from build123d import *

# Parameters (mm, degrees)
SALIENTE_EXTRUIR1_DEPTH    = 5
SALIENTE_EXTRUIR4_DEPTH    = 15
SALIENTE_EXTRUIR6_DEPTH    = 3
SALIENTE_EXTRUIR10_DEPTH   = 1
CROQUIS8_W                 = 24
CROQUIS8_H                 = 2
SALIENTE_EXTRUIR8_DEPTH    = 6
CROQUIS18_W                = 24
CROQUIS18_H                = 2
SALIENTE_EXTRUIR14_DEPTH   = 6
CROQUIS12_R                = 1.75
CORTAR_EXTRUIR1_DEPTH      = 29
CORTAR_EXTRUIR1_DEPTH_BACK = 3
CHAFL_N4_SIZE              = 7
CHAFL_N5_SIZE              = 10
REDONDEO1_R                = 3


with BuildPart() as part:
    # Croquis1 → Saliente-Extruir1 (new body)
    with BuildSketch(Plane.XY):
        with BuildLine():
            Line((0, 0), (24, 0))
            ThreePointArc((24, 0), (32, 8), (40, 0))
            Line((40, 0), (46, 0))
            Line((46, 0), (46, 12))
            Line((46, 12), (73, 12))
            Line((73, 12), (73, 0))
            Line((73, 0), (79, 0))
            Line((79, 0), (79, 30))
            Line((79, 30), (0, 30))
            Line((0, 30), (0, 0))
        make_face()
    extrude(amount=SALIENTE_EXTRUIR1_DEPTH)

    # Croquis4 → Saliente-Extruir4 (add)
    with BuildSketch(Plane.XY.offset(5)):
        Polygon((0, 30), (0, 0), (3, 0), (3, 27), (76, 27), (76, 0), (79, 0), (79, 30), align=None)
    extrude(amount=SALIENTE_EXTRUIR4_DEPTH)

    # Croquis6 → Saliente-Extruir6 (add)
    with BuildSketch(Plane.XY.offset(20)):
        with BuildLine():
            Line((0, 0), (0, 30))
            Line((0, 30), (79, 30))
            Line((79, 30), (79, 0))
            Line((79, 0), (40, 0))
            ThreePointArc((40, 0), (32, 8), (24, 0))
            Line((24, 0), (0, 0))
        make_face()
    extrude(amount=SALIENTE_EXTRUIR6_DEPTH)

    # Croquis13 → Saliente-Extruir10 (add)
    with BuildSketch(Plane(origin=(0, 0, 0), x_dir=(-1, 0, 0), z_dir=(0, 0, -1))):
        with BuildLine():
            Line((-79, 30), (-79, 0))
            Line((-79, 0), (-73, 0))
            Line((-73, 0), (-73, 12))
            Line((-73, 12), (-46, 12))
            Line((-46, 12), (-46, 0))
            Line((-46, 0), (-40, 0))
            Line((-40, 0), (-38, 0))
            ThreePointArc((-38, 0), (-32, 6), (-26, 0))
            Line((-26, 0), (0, 0))
            Line((0, 0), (0, 30))
            Line((0, 30), (-79, 30))
        make_face()
    extrude(amount=SALIENTE_EXTRUIR10_DEPTH)

    # Croquis8 → Saliente-Extruir8 (add)
    with BuildSketch(Plane(origin=(79, 0, 0), x_dir=(0, 0, -1), z_dir=(1, 0, 0))):
        with Locations((-11, 1)):
            Rectangle(CROQUIS8_W, CROQUIS8_H)
    extrude(amount=SALIENTE_EXTRUIR8_DEPTH)

    # Croquis18 → Saliente-Extruir14 (add)
    with BuildSketch(Plane.ZY):
        with Locations((11, 1)):
            Rectangle(CROQUIS18_W, CROQUIS18_H)
    extrude(amount=SALIENTE_EXTRUIR14_DEPTH)

    # Croquis12 → Cortar-Extruir1 (cut, two sides)
    with BuildSketch(Plane(origin=(0, 2, 0), x_dir=(1, 0, 0), z_dir=(0, 1, 0))) as cortar_extruir1_sk:
        with Locations((-3, -5)):
            Circle(CROQUIS12_R)
        with Locations((-3, -17)):
            Circle(CROQUIS12_R)
        with Locations((82, -17)):
            Circle(CROQUIS12_R)
        with Locations((82, -5)):
            Circle(CROQUIS12_R)
    extrude(amount=CORTAR_EXTRUIR1_DEPTH, mode=Mode.SUBTRACT)
    extrude(cortar_extruir1_sk.sketch, amount=-CORTAR_EXTRUIR1_DEPTH_BACK, mode=Mode.SUBTRACT)

    # Chaflán4
    chafl_n4_edges = [part.edges().sort_by_distance(p)[0] for p in [
        (3, 27, 12.5),
        (76, 27, 12.5),
    ]]
    chamfer(chafl_n4_edges, length=CHAFL_N4_SIZE)

    # Chaflán5
    chafl_n5_edges = [part.edges().sort_by_distance(p)[0] for p in [
        (0, 30, 11),
        (79, 30, 11),
    ]]
    chamfer(chafl_n5_edges, length=CHAFL_N5_SIZE)

    # Redondeo1
    redondeo1_edges = [part.edges().sort_by_distance(p)[0] for p in [
        (73, 12, 2),
        (46, 12, 2),
    ]]
    fillet(redondeo1_edges, radius=REDONDEO1_R)


solid = part.part
The listing builds one solid part. Answer for the finished solid, in the listing's coordinates (mm). A direction names the side the tool comes from. Coordinates: 2 decimals unless noted, no trailing zeros. Loops run counter-clockwise (first coordinate to the right, second up) from the corner with the lowest first, then second, coordinate; pieces in that order, holes last. Notation, with made-up numbers: (-3, 5) -> (18, 5) arc R17 cw to (18, 27) -> close; hole circle Ø10 at (41.5, 26.25). An arc over 180 degrees is marked (long way). Answer in a Markdown table with one row per item. Add a question column.
1. For faces 4 (the flat face through (85, 1, 11)), 5 (the flat face through (31, 17, 5)), 6 (the flat face through (79, 11, 11)), 7 (the cylindrical face through (32, 8, 2)), 8 (the flat face through (73, 4, 2)), determine the directions among +Z, -Z, +X, -X, +Y, -Y from which every point of the face is accessible in a straight line to the end or side of a thin tool.
2. Consider line 1 (Z direction, x = 82, y = 1.3); line 2 (Z direction, x = 16, y = 16.25); line 3 (X direction, y = 0.6, z = 17). Determine where each line is inside the solid, lowest interval first. Write a range as [from, to].
3. Flat-ended cylindrical pins translate along their axes: P1, Ø1.5, axis at x = 62.5, z = 19, coming from the -Y side; P2, Ø1, axis at x = 25.5, z = 5, coming from the -Y side; P3, Ø4.5, axis at y = 10.5, z = 11.5, coming from the +X side; P4, Ø2, axis at x = 82, z = 5, coming from the -Y side. Find the tip coordinate at first contact, or state that the pin passes through.
4. The part is cut by section B-B, the plane x = 82. Write down the section's boundary in (y, z).
5. Determine the mould class of faces 1 (the flat face through (43, 0, 2)), 2 (the flat face through (74, 25, 11)), 3 (the flat face through (60, 12, 2)) for opening direction X: +X half, -X half, draft (parallel to the pull), parting line (faces both ways), or undercut.
6. The part is cut by section C-C, the plane y = 17.75. Write down the section's boundary in (x, z).
7. The part is cut by section D-D, the plane x = 43. Write down the section's boundary in (y, z), then the cut area to 3 significant figures.
8. The part is cut by section A-A, the plane z = 17. Write down the section's boundary in (x, y).
Answer below:
| question | item | result |
|---|---|---|
| 1 | face 4 | +Z, -Z, +X, +Y, -Y |
| 1 | face 5 | -Y |
| 1 | face 6 | +Z, -Z, +X, +Y |
| 1 | face 7 | +Z, -Y |
| 1 | face 8 | -Z, -Y |
| 2 | line 1 | [-1, 3.25], [6.75, 15.25], [18.75, 23] |
| 2 | line 2 | [-1, 5], [20, 23] |
| 2 | line 3 | [-6, -4.75], [-1.25, 3], [76, 80.25], [83.75, 85] |
| 3 | P1 | y = 27 |
| 3 | P2 | y = 3.87 |
| 3 | P3 | x = 79 |
| 3 | P4 | through |
| 4 | outline | (0, -1) -> (2, -1) -> (2, 3.25) -> (0, 3.25) -> close; (0, 6.75) -> (2, 6.75) -> (2, 15.25) -> (0, 15.25) -> close; (0, 18.75) -> (2, 18.75) -> (2, 23) -> (0, 23) -> close |
| 5 | face 1 | draft |
| 5 | face 2 | +X half |
| 5 | face 3 | undercut |
| 6 | outline | (0, -1) -> (79, -1) -> (79, 23) -> (0, 23) -> close; hole (3, 5) -> (76, 5) -> (76, 20) -> (3, 20) -> close |
| 7 | outline | (0, -1) -> (30, -1) -> (30, 23) -> (0, 23) -> (0, 20) -> (27, 20) -> (27, 5) -> (0, 5) -> close |
| 7 | area | 315 mm2 |
| 8 | outline | (-6, 0) -> (-4.75, 0) -> (-4.75, 2) -> (-6, 2) -> close; (-1.25, 0) -> (3, 0) -> (3, 20) -> (10, 27) -> (69, 27) -> (76, 20) -> (76, 0) -> (80.25, 0) -> (80.25, 2) -> (79, 2) -> (79, 20) -> (69, 30) -> (10, 30) -> (0, 20) -> (0, 2) -> (-1.25, 2) -> close; (83.75, 0) -> (85, 0) -> (85, 2) -> (83.75, 2) -> close |
